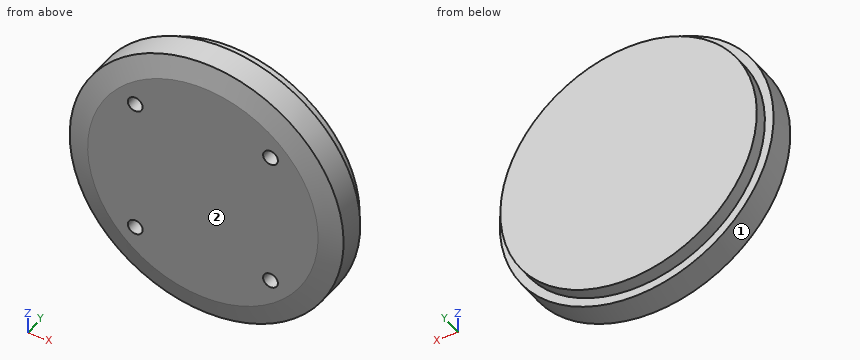
from build123d import *

# Parameters (mm, degrees)
M3_CLEARANCE_HOLE1_D     = 3.4
M3_CLEARANCE_HOLE1_DEPTH = 4
M3_CLEARANCE_HOLE1_TIP   = 1.021463052
SKETCH5_R                = 29.5
BOSS_EXTRUDE1_DEPTH      = 3


with BuildPart() as part:
    # Sketch1 → Revolve1 (revolve)
    with BuildSketch(Plane.XY, mode=Mode.PRIVATE) as revolve1_sk:
        Polygon((-26.5, -7.6), (-31.5, -6.2), (-31.5, 0), (0, 0), (0, -7.6), align=None)
    revolve(revolve1_sk.sketch.rotate(Axis((0, -13.2, 0), (0, 1, 0)), 270), axis=Axis((0, -13.2, 0), (0, 1, 0)))

    # M3 Clearance Hole1
    with Locations(Plane(origin=(0, -7.6, 0), x_dir=(-1, 0, 0), z_dir=(0, -1, 0))):
        with Locations((15.556349186, -15.556349186), (15.556349186, 15.556349186), (-15.556349186, 15.556349186), (-15.556349186, -15.556349186)):
            Hole(M3_CLEARANCE_HOLE1_D / 2, depth=M3_CLEARANCE_HOLE1_DEPTH)
            with Locations((0, 0, -(M3_CLEARANCE_HOLE1_DEPTH + M3_CLEARANCE_HOLE1_TIP / 2))):  # 118° drill point
                Cone(0, M3_CLEARANCE_HOLE1_D / 2, M3_CLEARANCE_HOLE1_TIP, mode=Mode.SUBTRACT)

    # Sketch5 → Boss-Extrude1 (add)
    with BuildSketch(Plane(origin=(0, 0, 0), x_dir=(1, 0, 0), z_dir=(0, 1, 0))):
        with Locations(Location((0, 0, 0), (0, 0, 270))):
            Circle(SKETCH5_R)
    extrude(amount=BOSS_EXTRUDE1_DEPTH)


solid = part.part
Can you work these out from the model? Positions are in its coordinate system, mm. Face numbers are marked on the shaded views. Round coordinates to 2 decimals unless told otherwise and drop trailing zeros. Loops run counter-clockwise (first coordinate to the right, second up) from the corner with the lowest first, then second, coordinate; pieces in that order, holes last. Notation, with made-up numbers: (-15.75, 69.25) - (32.25, 69.25) arc R20 cw to (32.25, 83.25) - close; hole circle Ø5 at (-21, 58.5). An arc over 180 degrees is marked (long way). Write item = value, one per line. Start each with the question number.
(1) If I drill on probe 1 along X at (y, z) = (-3.5, -16.5); probe 2 along Z at (x, y) = (-7, -4.5); probe 3 along Z at (x, y) = (-5.5, -1.75), over which ranges is the centre line in solid material (lowest first)? Write a range as [from, to].
(2) For P1, Ø2, axis at x = 11, y = -3, coming from the +Z side; P2, Ø3, axis at x = 15.56, z = 15.56, coming from the -Y side, each with a flat end and sliding along its axis, tell me the tip position at first contact or that it passes through.
(3) If we mould it in two halves opening along Z, with no side actions, what happens to the marked faces 1 and 2? For each: released by +Z, released by -Z, zero draft, split by the parting line, or undercut.
(4) If we section it at A-A (z = 0): Please give me the cut outline in (x, y), and give its area (3 significant figures).
(5) If we section it at B-B (x = 0): Please give me the cut outline in (y, z), and give its area (3 significant figures).
(6) If we section it at C-C (y = 1.25): Please give me the cut outline in (x, z).
Ans:
q1.probe_1 = [-26.83, -16.77], [-14.35, 14.35], [16.77, 26.83]
q1.probe_2 = [-30.71, 30.71]
q1.probe_3 = [-31.02, 31.02]
q2.P1 = 29.87
q2.P2 = -3.48
q3.face_1 = split by the parting line
q3.face_2 = zero draft
q4.outline = (-31.5, -6.2) - (-26.5, -7.6) - (26.5, -7.6) - (31.5, -6.2) - (31.5, 0) - (29.5, 0) - (29.5, 3) - (-29.5, 3) - (-29.5, 0) - (-31.5, 0) - close
q4.area = 649 mm²
q5.outline = (-7.6, -26.5) - (-6.2, -31.5) - (0, -31.5) - (0, -29.5) - (3, -29.5) - (3, 29.5) - (0, 29.5) - (0, 31.5) - (-6.2, 31.5) - (-7.6, 26.5) - close
q5.area = 649 mm²
q6.outline = circle Ø59 at (0, 0)
